Part model, mm, in its own coordinate system. A direction names the side the tool comes from. Round coordinates to 2 decimals unless told otherwise and drop trailing zeros. Loops run counter-clockwise (first coordinate to the right, second up) from the corner with the lowest first, then second, coordinate; pieces in that order, holes last.
(1) Cut at D-D on z = -15. List the corners of the cut face in (x, y).
(2) Tool access for faces 1 (the face through (0, 50, 27)), 2 (the face through (-1, 35, -25)), 3 (the face through (7.509, 64.93, 23.846)), 4 (the face through (20.81, 74.93, 21.61)), 5 (the face through (-1, 25, 25)): list every direction of +Z, -Z, +X, -X, +Y, -Y with a clear straight run to the whole face (end or side of a thin tool).
(3) Mould opens along X. For faces 6 (the face through (-75, 26, 0)), 7 (the face through (75, 27, 0)), 8 (the face through (-45.79, 26.55, 30.42)) say: +X half, -X half, draft (parallel to the pull), parting line (faces both ways), or undercut.
(4) Flat gauge pins, fed straight in: pin 1 (3 mm diameter, centred on x = 60.06, y = 31.46, fed in from -Z); pin 2 (1 mm diameter, centred on x = -7.5, y = 9, fed in from +Z) (3 decimals); pin 3 (10 mm diameter, centred on x = -36, z = -11, fed in from -Y). Where does each tip first touch, or does it go through?
(5) Probe probe 1 along Y at (x, z) = (-5, 28); probe 2 along Z at (x, y) = (-64.5, 34.5); probe 3 along Z at (x, y) = (7, 38). List the from-to ranges inside material, lowest first.
(6) Cut at A-A on x = -55. List the corners of the cut face in (y, z), then the cut area to 3 significant figures.
(7) Cut at B-B on z = 0. List the corners of the cut face in (x, y).
(8) Cut at C-C on y = 13. List the corners of the cut face in (x, z).
from build123d import *

# Parameters (mm, degrees)
SKIZZE1_W                       = 150
SKIZZE1_H                       = 50
AUFSATZ_LINEAR_AUSTRAGEN1_DEPTH = 50
SKIZZE2_R                       = 10
AUFSATZ_LINEAR_AUSTRAGEN2_DEPTH = 150
SCHNITT_LINEAR_AUSTRAGEN1_DEPTH = 182
SKIZZE4_R                       = 12.5
SKIZZE4_R_2                     = 10
SKIZZE4_R_3                     = 1
SKIZZE4_R_4                     = 7.5
AUFSATZ_LINEAR_AUSTRAGEN3_DEPTH = 11
SKIZZE5_R                       = 30
AUFSATZ_LINEAR_AUSTRAGEN4_DEPTH = 30
SCHNITT_LINEAR_START            = -20
SKIZZE6_R                       = 30
SKIZZE6_R_2                     = 25
SCHNITT_LINEAR_AUSTRAGEN3_DEPTH = 10


with BuildPart() as part:
    # Skizze1 → Aufsatz-Linear austragen1 (new body)
    with BuildSketch(Plane(origin=(0, 0, 0), x_dir=(1, 0, 0), z_dir=(0, 1, 0))):
        Rectangle(SKIZZE1_W, SKIZZE1_H)
    extrude(amount=AUFSATZ_LINEAR_AUSTRAGEN1_DEPTH)

    # Skizze2 → Aufsatz-Linear austragen2 (add)
    with BuildSketch(Plane(origin=(75, 0, 0), x_dir=(0, 0, -1), z_dir=(1, 0, 0))):
        Circle(SKIZZE2_R)
    extrude(amount=-AUFSATZ_LINEAR_AUSTRAGEN2_DEPTH)

    # Skizze3 → Schnitt-Linear austragen1 (cut)
    with BuildSketch(Plane(origin=(75, 0, 0), x_dir=(0, 0, -1), z_dir=(1, 0, 0))):
        Polygon((-10, 0), (-25, 20), (-25, 0), align=None)
        Polygon((25, 20), (25, 0), (10, 0), align=None)
    extrude(amount=-SCHNITT_LINEAR_AUSTRAGEN1_DEPTH, mode=Mode.SUBTRACT)

    # Skizze4 → Aufsatz-Linear austragen3 (add)
    # profile 1 of 3: a face of its own
    with BuildSketch(Plane.XY.offset(25)):
        with Locations(Location((-55, 35, 0), (0, 0, 180))):
            Circle(SKIZZE4_R)
    # profile 2 of 3: a face of its own
    with BuildSketch(Plane.XY.offset(25)):
        with Locations(Location((56.52620572, 35, 0), (0, 0, 180))):
            Circle(SKIZZE4_R_2)
        with Locations((56.52620572, 40)):
            Circle(SKIZZE4_R_3, mode=Mode.SUBTRACT)
        with Locations((60.061739626, 38.535533906)):
            Circle(SKIZZE4_R_3, mode=Mode.SUBTRACT)
        with Locations((61.52620572, 35)):
            Circle(SKIZZE4_R_3, mode=Mode.SUBTRACT)
        with Locations((60.061739626, 31.464466094)):
            Circle(SKIZZE4_R_3, mode=Mode.SUBTRACT)
        with Locations((56.52620572, 30)):
            Circle(SKIZZE4_R_3, mode=Mode.SUBTRACT)
        with Locations((52.990671814, 31.464466094)):
            Circle(SKIZZE4_R_3, mode=Mode.SUBTRACT)
        with Locations((51.52620572, 35)):
            Circle(SKIZZE4_R_3, mode=Mode.SUBTRACT)
        with Locations((52.990671814, 38.535533906)):
            Circle(SKIZZE4_R_3, mode=Mode.SUBTRACT)
    # profile 3 of 3: a face of its own
    with BuildSketch(Plane.XY.offset(25)):
        with Locations(Location((0, 35, 0), (0, 0, 180))):
            Circle(SKIZZE4_R_4)
        with Locations((0, 38.75)):
            Circle(SKIZZE4_R_3, mode=Mode.SUBTRACT)
        with Locations((3.535533906, 38.535533906)):
            Circle(SKIZZE4_R_3, mode=Mode.SUBTRACT)
        with Locations((5, 35)):
            Circle(SKIZZE4_R_3, mode=Mode.SUBTRACT)
        with Locations((3.535533906, 31.464466094)):
            Circle(SKIZZE4_R_3, mode=Mode.SUBTRACT)
        with Locations((0, 30)):
            Circle(SKIZZE4_R_3, mode=Mode.SUBTRACT)
        with Locations((-3.535533906, 31.464466094)):
            Circle(SKIZZE4_R_3, mode=Mode.SUBTRACT)
        with Locations((-5, 35)):
            Circle(SKIZZE4_R_3, mode=Mode.SUBTRACT)
        with Locations((-3.535533906, 38.535533906)):
            Circle(SKIZZE4_R_3, mode=Mode.SUBTRACT)
    extrude(amount=AUFSATZ_LINEAR_AUSTRAGEN3_DEPTH)

    # Skizze5 → Aufsatz-Linear austragen4 (add)
    with BuildSketch(Plane(origin=(0, 50, 0), x_dir=(1, 0, 0), z_dir=(0, 1, 0))):
        with Locations(Location((0, 0, 0), (0, 0, 56.442690238))):
            Circle(SKIZZE5_R)
    extrude(amount=AUFSATZ_LINEAR_AUSTRAGEN4_DEPTH)

    # Skizze6 → Schnitt-Linear austragen3 (cut)
    with BuildSketch(Plane(origin=(0, 80, 0), x_dir=(1, 0, 0), z_dir=(0, 1, 0)).offset(SCHNITT_LINEAR_START)):
        with Locations(Location((0, 0, 0), (0, 0, 56.442690238))):
            Circle(SKIZZE6_R)
        with Locations(Location((0, 0, 0), (0, 0, 270))):
            Circle(SKIZZE6_R_2, mode=Mode.SUBTRACT)
    extrude(amount=SCHNITT_LINEAR_AUSTRAGEN3_DEPTH, mode=Mode.SUBTRACT)


solid = part.part
Final values:
1. outline: (-75, 6.67) - (75, 6.67) - (75, 50) - (25.98, 50) - (25.98, 60) - (20, 60) - (20, 70) - (25.98, 70) - (25.98, 80) - (-25.98, 80) - (-25.98, 70) - (-20, 70) - (-20, 60) - (-25.98, 60) - (-25.98, 50) - (-75, 50) - close
2. face 1: +Z, +X, -X
2. face 2: -Z, +X, -X, -Y
2. face 3: none
2. face 4: +Y
2. face 5: +Z
3. face 6: -X half
3. face 7: +X half
3. face 8: undercut
4. pin 1: stops at z = -25
4. pin 2: stops at z = 17.125
4. pin 3: stops at y = -8
5. probe 1: y = 29.41 to 34, 36 to 40.59, 50 to 60, 70 to 80
5. probe 2: z = -25 to 36
5. probe 3: z = -25 to 25
6. outline: (0, -10) - (20, -25) - (50, -25) - (50, 25) - (47.5, 25) - (47.5, 36) - (22.5, 36) - (22.5, 25) - (20, 25) - (0, 10) arc R10 ccw to start
6. area: 2,630 mm2
7. outline: (-75, -10) - (75, -10) - (75, 50) - (30, 50) - (30, 60) - (25, 60) - (25, 70) - (30, 70) - (30, 80) - (-30, 80) - (-30, 70) - (-25, 70) - (-25, 60) - (-30, 60) - (-30, 50) - (-75, 50) - close
8. outline: (-75, -19.75) - (75, -19.75) - (75, 19.75) - (-75, 19.75) - close
